from build123d import *

# Parameters (mm, degrees)
SKETCH_1_R      = 2.5
EXTRUDE_1_DEPTH = 100


with BuildPart() as part:
    # 草图1 → 凸台-拉伸1 (new body)
    with BuildSketch(Plane.XY):
        with BuildLine():
            Line((-11.580766307, 11.574521058), (-11.580766307, 4.474521058))
            ThreePointArc((-11.580766307, 4.474521058), (-11.492898341, 4.262389024), (-11.280766307, 4.174521058))
            Line((-11.280766307, 4.174521058), (-11.080766307, 4.174521058))
            Line((-11.080766307, 4.174521058), (-11.080766307, 3.974521058))
            ThreePointArc((-11.080766307, 3.974521058), (-10.992898341, 3.762389024), (-10.780766307, 3.674521058))
            Line((-10.780766307, 3.674521058), (-9.880766307, 3.674521058))
            ThreePointArc((-9.880766307, 3.674521058), (-9.668634272, 3.762389024), (-9.580766307, 3.974521058))
            Line((-9.580766307, 3.974521058), (-9.580766307, 7.774521058))
            ThreePointArc((-9.580766307, 7.774521058), (-9.492898341, 7.986653093), (-9.280766307, 8.074521058))
            Line((-9.280766307, 8.074521058), (-8.409193431, 8.074521058))
            ThreePointArc((-8.409193431, 8.074521058), (-8.026509999, 7.998400591), (-7.70208665, 7.78162784))
            Line((-7.70208665, 7.78162784), (-4.273659525, 4.353200715))
            ThreePointArc((-4.273659525, 4.353200715), (-4.056886774, 4.028777366), (-3.980766307, 3.646093934))
            Line((-3.980766307, 3.646093934), (-3.980766307, -2.497051817))
            ThreePointArc((-3.980766307, -2.497051817), (-4.056886774, -2.879735249), (-4.273659525, -3.204158598))
            Line((-4.273659525, -3.204158598), (-7.70208665, -6.632585723))
            ThreePointArc((-7.70208665, -6.632585723), (-8.026509999, -6.849358474), (-8.409193431, -6.925478942))
            Line((-8.409193431, -6.925478942), (-9.280766307, -6.925478942))
            ThreePointArc((-9.280766307, -6.925478942), (-9.492898341, -6.837610976), (-9.580766307, -6.625478942))
            Line((-9.580766307, -6.625478942), (-9.580766307, -2.825478942))
            ThreePointArc((-9.580766307, -2.825478942), (-9.668634272, -2.613346907), (-9.880766307, -2.525478942))
            Line((-9.880766307, -2.525478942), (-10.780766307, -2.525478942))
            ThreePointArc((-10.780766307, -2.525478942), (-10.992898341, -2.613346907), (-11.080766307, -2.825478942))
            Line((-11.080766307, -2.825478942), (-11.080766307, -3.025478942))
            Line((-11.080766307, -3.025478942), (-11.280766307, -3.025478942))
            ThreePointArc((-11.280766307, -3.025478942), (-11.492898341, -3.113346907), (-11.580766307, -3.325478942))
            Line((-11.580766307, -3.325478942), (-11.580766307, -10.425478942))
            ThreePointArc((-11.580766307, -10.425478942), (-11.141426478, -11.486139113), (-10.080766307, -11.925478942))
            Line((-10.080766307, -11.925478942), (-2.980766307, -11.925478942))
            ThreePointArc((-2.980766307, -11.925478942), (-2.768634272, -11.837610976), (-2.680766307, -11.625478942))
            Line((-2.680766307, -11.625478942), (-2.680766307, -11.425478942))
            Line((-2.680766307, -11.425478942), (-2.480766307, -11.425478942))
            ThreePointArc((-2.480766307, -11.425478942), (-2.268634272, -11.337610976), (-2.180766307, -11.125478942))
            Line((-2.180766307, -11.125478942), (-2.180766307, -10.225478942))
            ThreePointArc((-2.180766307, -10.225478942), (-2.268634272, -10.013346907), (-2.480766307, -9.925478942))
            Line((-2.480766307, -9.925478942), (-6.280766307, -9.925478942))
            ThreePointArc((-6.280766307, -9.925478942), (-6.492898341, -9.837610976), (-6.580766307, -9.625478942))
            Line((-6.580766307, -9.625478942), (-6.580766307, -8.753906066))
            ThreePointArc((-6.580766307, -8.753906066), (-6.504645839, -8.371222634), (-6.287873088, -8.046799285))
            Line((-6.287873088, -8.046799285), (-2.859445963, -4.61837216))
            ThreePointArc((-2.859445963, -4.61837216), (-2.535022614, -4.401599409), (-2.152339182, -4.325478942))
            Line((-2.152339182, -4.325478942), (3.990806569, -4.325478942))
            ThreePointArc((3.990806569, -4.325478942), (4.373490001, -4.401599409), (4.69791335, -4.61837216))
            Line((4.69791335, -4.61837216), (8.126340475, -8.046799285))
            ThreePointArc((8.126340475, -8.046799285), (8.343113226, -8.371222634), (8.419233693, -8.753906066))
            Line((8.419233693, -8.753906066), (8.419233693, -9.625478942))
            ThreePointArc((8.419233693, -9.625478942), (8.331365728, -9.837610976), (8.119233693, -9.925478942))
            Line((8.119233693, -9.925478942), (4.319233693, -9.925478942))
            ThreePointArc((4.319233693, -9.925478942), (4.107101659, -10.013346907), (4.019233693, -10.225478942))
            Line((4.019233693, -10.225478942), (4.019233693, -11.125478942))
            ThreePointArc((4.019233693, -11.125478942), (4.107101659, -11.337610976), (4.319233693, -11.425478942))
            Line((4.319233693, -11.425478942), (4.519233693, -11.425478942))
            Line((4.519233693, -11.425478942), (4.519233693, -11.625478942))
            ThreePointArc((4.519233693, -11.625478942), (4.607101659, -11.837610976), (4.819233693, -11.925478942))
            Line((4.819233693, -11.925478942), (11.919233693, -11.925478942))
            ThreePointArc((11.919233693, -11.925478942), (12.979893865, -11.486139113), (13.419233693, -10.425478942))
            Line((13.419233693, -10.425478942), (13.419233693, -3.325478942))
            ThreePointArc((13.419233693, -3.325478942), (13.331365728, -3.113346907), (13.119233693, -3.025478942))
            Line((13.119233693, -3.025478942), (12.919233693, -3.025478942))
            Line((12.919233693, -3.025478942), (12.919233693, -2.825478942))
            ThreePointArc((12.919233693, -2.825478942), (12.831365728, -2.613346907), (12.619233693, -2.525478942))
            Line((12.619233693, -2.525478942), (11.719233693, -2.525478942))
            ThreePointArc((11.719233693, -2.525478942), (11.507101659, -2.613346907), (11.419233693, -2.825478942))
            Line((11.419233693, -2.825478942), (11.419233693, -6.625478942))
            ThreePointArc((11.419233693, -6.625478942), (11.331365728, -6.837610976), (11.119233693, -6.925478942))
            Line((11.119233693, -6.925478942), (10.247660818, -6.925478942))
            ThreePointArc((10.247660818, -6.925478942), (9.864977386, -6.849358474), (9.540554037, -6.632585723))
            Line((9.540554037, -6.632585723), (6.112126912, -3.204158598))
            ThreePointArc((6.112126912, -3.204158598), (5.895354161, -2.879735249), (5.819233693, -2.497051817))
            Line((5.819233693, -2.497051817), (5.819233693, 3.646093934))
            ThreePointArc((5.819233693, 3.646093934), (5.895354161, 4.028777366), (6.112126912, 4.353200715))
            Line((6.112126912, 4.353200715), (9.540554037, 7.78162784))
            ThreePointArc((9.540554037, 7.78162784), (9.864977386, 7.998400591), (10.247660818, 8.074521058))
            Line((10.247660818, 8.074521058), (11.119233693, 8.074521058))
            ThreePointArc((11.119233693, 8.074521058), (11.331365728, 7.986653093), (11.419233693, 7.774521058))
            Line((11.419233693, 7.774521058), (11.419233693, 3.974521058))
            ThreePointArc((11.419233693, 3.974521058), (11.507101659, 3.762389024), (11.719233693, 3.674521058))
            Line((11.719233693, 3.674521058), (12.619233693, 3.674521058))
            ThreePointArc((12.619233693, 3.674521058), (12.831365728, 3.762389024), (12.919233693, 3.974521058))
            Line((12.919233693, 3.974521058), (12.919233693, 4.174521058))
            Line((12.919233693, 4.174521058), (13.119233693, 4.174521058))
            ThreePointArc((13.119233693, 4.174521058), (13.331365728, 4.262389024), (13.419233693, 4.474521058))
            Line((13.419233693, 4.474521058), (13.419233693, 11.574521058))
            ThreePointArc((13.419233693, 11.574521058), (12.979893865, 12.63518123), (11.919233693, 13.074521058))
            Line((11.919233693, 13.074521058), (4.819233693, 13.074521058))
            ThreePointArc((4.819233693, 13.074521058), (4.607101659, 12.986653093), (4.519233693, 12.774521058))
            Line((4.519233693, 12.774521058), (4.519233693, 12.574521058))
            Line((4.519233693, 12.574521058), (4.319233693, 12.574521058))
            ThreePointArc((4.319233693, 12.574521058), (4.107101659, 12.486653093), (4.019233693, 12.274521058))
            Line((4.019233693, 12.274521058), (4.019233693, 11.374521058))
            ThreePointArc((4.019233693, 11.374521058), (4.107101659, 11.162389024), (4.319233693, 11.074521058))
            Line((4.319233693, 11.074521058), (8.119233693, 11.074521058))
            ThreePointArc((8.119233693, 11.074521058), (8.331365728, 10.986653093), (8.419233693, 10.774521058))
            Line((8.419233693, 10.774521058), (8.419233693, 9.902948183))
            ThreePointArc((8.419233693, 9.902948183), (8.343113226, 9.520264751), (8.126340475, 9.195841402))
            Line((8.126340475, 9.195841402), (4.69791335, 5.767414277))
            ThreePointArc((4.69791335, 5.767414277), (4.373490001, 5.550641526), (3.990806569, 5.474521058))
            Line((3.990806569, 5.474521058), (-2.152339182, 5.474521058))
            ThreePointArc((-2.152339182, 5.474521058), (-2.535022614, 5.550641526), (-2.859445963, 5.767414277))
            Line((-2.859445963, 5.767414277), (-6.287873088, 9.195841402))
            ThreePointArc((-6.287873088, 9.195841402), (-6.504645839, 9.520264751), (-6.580766307, 9.902948183))
            Line((-6.580766307, 9.902948183), (-6.580766307, 10.774521058))
            ThreePointArc((-6.580766307, 10.774521058), (-6.492898341, 10.986653093), (-6.280766307, 11.074521058))
            Line((-6.280766307, 11.074521058), (-2.480766307, 11.074521058))
            ThreePointArc((-2.480766307, 11.074521058), (-2.268634272, 11.162389024), (-2.180766307, 11.374521058))
            Line((-2.180766307, 11.374521058), (-2.180766307, 12.274521058))
            ThreePointArc((-2.180766307, 12.274521058), (-2.268634272, 12.486653093), (-2.480766307, 12.574521058))
            Line((-2.480766307, 12.574521058), (-2.680766307, 12.574521058))
            Line((-2.680766307, 12.574521058), (-2.680766307, 12.774521058))
            ThreePointArc((-2.680766307, 12.774521058), (-2.768634272, 12.986653093), (-2.980766307, 13.074521058))
            Line((-2.980766307, 13.074521058), (-10.080766307, 13.074521058))
            ThreePointArc((-10.080766307, 13.074521058), (-11.141426478, 12.63518123), (-11.580766307, 11.574521058))
        make_face()
        with Locations((0.919233693, 0.574521058)):
            Circle(SKETCH_1_R, mode=Mode.SUBTRACT)
    extrude(amount=EXTRUDE_1_DEPTH)


solid = part.part
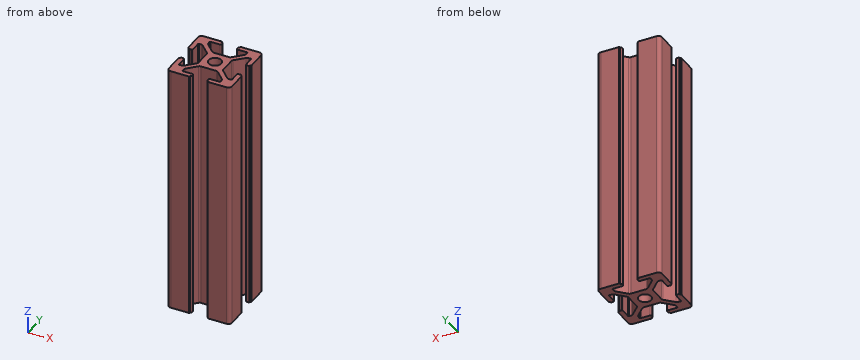
Model file for the job. Use its own axes, mm. Give positions to 0.01 mm unless a question says otherwise; leave off trailing zeros. Loops run counter-clockwise (first coordinate to the right, second up) from the corner with the lowest first, then second, coordinate; pieces in that order, holes last. Notation, with made-up numbers: (-20.5, 8) -> (23.5, 8) arc R18 ccw to (23.5, 37) -> close; hole circle Ø7 at (15, 70.25). An arc over 180 degrees is marked (long way). Use a Markdown table: item, result. Add a question column.
(1) Wall check: line 1 along X through (y, z) = (-4.5, 93.5); line 2 along X through (y, z) = (7.75, 66.5); line 3 along Y through (x, z) = (1, 92). Give the ranges that are in metal, low to high.
(2) Drop flat-ended pins along their axis: pin 1 Ø10 at (x, y) = (6.5, -4.5) entering from -Z; pin 2 Ø1.8 at (y, z) = (1, 39.5) entering from +X; pin 3 Ø1.5 at (x, z) = (-1, 63.5) entering from +Y; pin 4 Ø1 at (x, z) = (2, 72.5) entering from -Y. Give the stop position or say it passes through.
(3) Slice it at B-B on x = -5.25. List the corners of the cut face in (y, z), and give its area (3 significant figures).
(4) Slice it at A-A on x = 1.5. List the corners of the cut face in (y, z), and give its area (3 significant figures).
Filled sheet:
| question | item | result |
|---|---|---|
| 1 | line 1 | -11.58 to -9.58, -5.57 to -2.72, 4.56 to 7.41, 11.42 to 13.42 |
| 1 | line 2 | -11.58 to -9.58, -7.67 to -4.84, 6.68 to 9.51, 11.42 to 13.42 |
| 1 | line 3 | -4.33 to -1.92, 3.07 to 5.47 |
| 2 | pin 1 | z = 0 |
| 2 | pin 2 | x = 5.82 |
| 2 | pin 3 | y = 5.47 |
| 2 | pin 4 | y = -4.33 |
| 3 | outline | (-11.93, 0) -> (-9.93, 0) -> (-9.93, 100) -> (-11.93, 100) -> close; (-7.01, 0) -> (-4.18, 0) -> (-4.18, 100) -> (-7.01, 100) -> close; (5.33, 0) -> (8.16, 0) -> (8.16, 100) -> (5.33, 100) -> close; (11.07, 0) -> (13.07, 0) -> (13.07, 100) -> (11.07, 100) -> close |
| 3 | area | 966 mm2 |
| 4 | outline | (-4.33, 0) -> (-1.86, 0) -> (-1.86, 100) -> (-4.33, 100) -> close; (3.01, 0) -> (5.47, 0) -> (5.47, 100) -> (3.01, 100) -> close |
| 4 | area | 494 mm2 |
